Here's the drawing with two shaded views (mm, measured from the low corner). I have some questions. A direction names the side the tool comes from. Round coordinates to 2 decimals unless told otherwise and drop trailing zeros. Write each loop counter-clockwise with the first axis right and the second up, starting at its lowest first coordinate (ties: lowest second). Pieces come first, ordered by that corner, then holes.
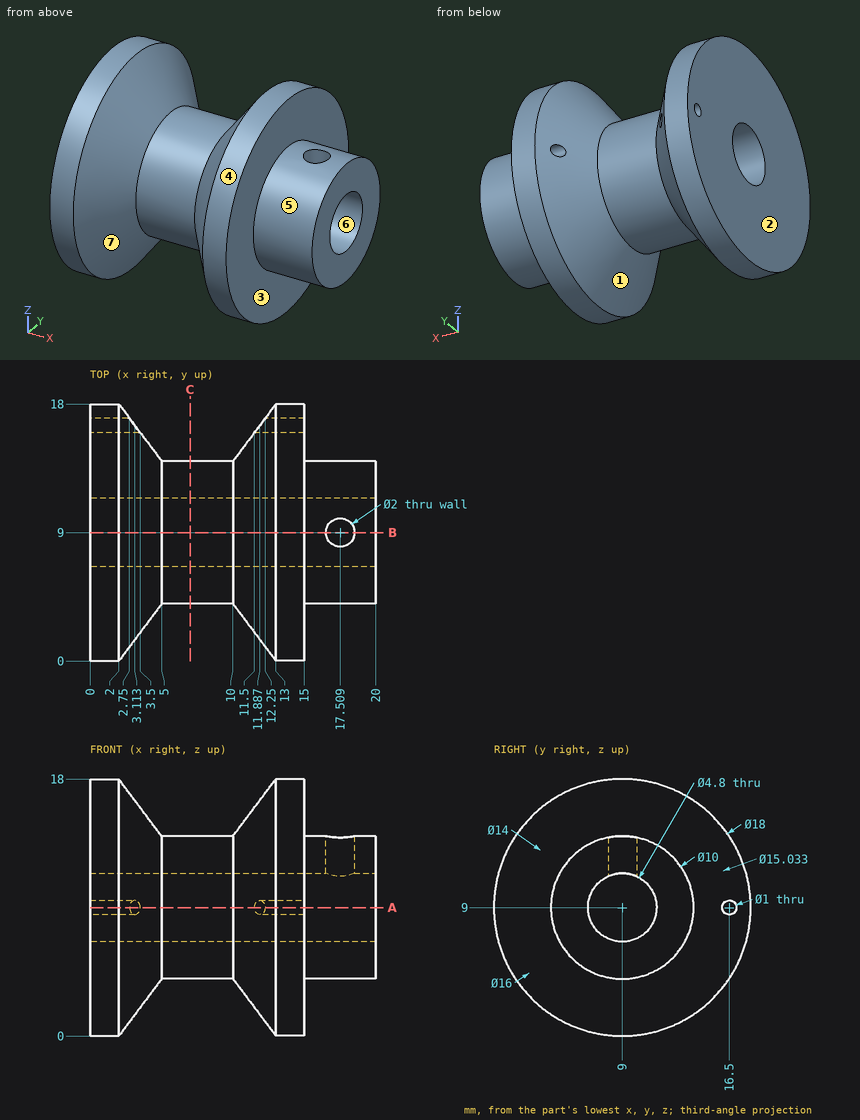
Q1. Imagine slicing it at A-A, the plane z = 9. Write out the boundary of the cut face in (x, y), then the cut area to 3 significant figures.
Q2. If I drill on L1, parallel to X at y = 2.5, z = 10.5 (1 decimal); L2, parallel to X at y = 12, z = 16.25 (1 decimal); L3, parallel to Y at x = 7.25, z = 9.75 (1 decimal), over which ranges is the centre line in solid material (lowest first)?
Q3. Imagine slicing it at B-B, the plane y = 9. Write out the boundary of the cut face in (x, z), then the cut area to 3 significant figures.
Q4. We'd pull the mould along X, two halves only. Please class the marked faces 1, 2, 3 and 4: pulls with the +X half, pulls with the -X half, needs draft (parallel to the pull), parting line crosses it, or undercut.
Q5. Imagine slicing it at C-C, the plane x = 7. Write out the boundary of the cut face in (y, z).
Q6. I'm going to push flat-ended pins straight in: pin 1 Ø4 at (x, z) = (16.5, 10) entering from -Y; pin 2 Ø4 at (x, y) = (6, 4.5) entering from -Z (1 decimal); pin 3 Ø4 at (x, y) = (11.5, 4.5) entering from +Z; pin 4 Ø5 at (x, z) = (13.5, 3) entering from +Y. Where does each tip first touch, or does it pass through?
Q7. On a 3-axis mill with a long thin cutter (end or side, diameter ignored), from which of +Z, -Z, +X, -X, +Y, -Y can I reach the whole of each face in a straight line? I mean the marked faces 5, 6 and 7. Say none if no direction works.
Results found:
1. outline: (0, 0) - (2, 0) - (5, 4) - (10, 4) - (13, 0) - (15, 0) - (15, 4) - (20, 4) - (20, 6.6) - (0, 6.6) - close; (0, 11.4) - (20, 11.4) - (20, 14) - (15, 14) - (15, 16) - (11.5, 16) - (10, 14) - (5, 14) - (3.5, 16) - (0, 16) - close; (0, 17) - (2.75, 17) - (2, 18) - (0, 18) - close; (12.25, 17) - (15, 17) - (15, 18) - (13, 18) - close
1. area: 154 mm2
2. L1: x = 0 to 3.7, 11.3 to 15
2. L2: x = 0 to 2.9, 12.1 to 15
2. L3: y = 4.1 to 6.7, 11.3 to 13.9
3. outline: (0, 0) - (2, 0) - (5, 4) - (10, 4) - (13, 0) - (15, 0) - (15, 4) - (20, 4) - (20, 6.6) - (0, 6.6) - close; (0, 11.4) - (16.51, 11.4) - (16.51, 14) - (15, 14) - (15, 18) - (13, 18) - (10, 14) - (5, 14) - (2, 18) - (0, 18) - close; (18.51, 11.4) - (20, 11.4) - (20, 14) - (18.51, 14) - close
3. area: 155 mm2
4. face 1: undercut
4. face 2: pulls with the -X half
4. face 3: pulls with the +X half
4. face 4: needs draft
5. outline: circle Ø10 at (9, 9); hole circle Ø4.8 at (9, 9)
6. pin 1: stops at y = 0
6. pin 2: stops at z = 4.1
6. pin 3: stops at z = 17.42
6. pin 4: stops at y = 17.29
7. face 5: +X
7. face 6: +X, -X
7. face 7: none
